```python
from build123d import *

# Parameters (mm, degrees)
F0_R     = 20
F1_DEPTH = 6
F2_R     = 5
F3_DEPTH = 12
F4_R     = 2.75
F5_DEPTH = 18.001
F6_R     = 5
F7_DEPTH = 5


with BuildPart() as f1:
    # F0 (on Top) → F1 (new body)
    with BuildSketch(Plane.XY):
        Circle(F0_R)
    extrude(amount=F1_DEPTH)

    # F2 (on face) → F3 (join)
    with BuildSketch(Plane.XY.offset(6)):
        Circle(F2_R)
    extrude(amount=F3_DEPTH)

    # F4 (on face) → F5 (cut, through all)
    with BuildSketch(Plane.XY.offset(18)):
        Circle(F4_R)
    extrude(amount=-F5_DEPTH, mode=Mode.SUBTRACT)

    # F6 (on face) → F7 (cut)
    with BuildSketch(Plane.XY):
        Circle(F6_R)
    extrude(amount=F7_DEPTH, mode=Mode.SUBTRACT)


solid = f1.part
```
Check sheet for the modelled part. Datum: model origin and axes. Units: mm. A direction names the side the tool comes from. Coordinates: 2 decimals unless noted, no trailing zeros. Write each loop counter-clockwise with the first axis right and the second up, starting at its lowest first coordinate (ties: lowest second). Pieces come first, ordered by that corner, then holes. Notation, with made-up numbers: M 3.5,34.25 L 50.5,34.25 A21 cw 50.5,43.25 Z; hole C 66,-9 d7. An arc over 180 degrees is marked long. Write item = value, one per line. Start each with the question number.
1. Mould release check, pull along Y, two halves, no side actions. Record for faces 3 (the flat face through (2.2, -2.2, 18)), 4 (the cylindrical face through (-1.08, -4.88, 2.46)), 5 (the cylindrical face through (-1.08, -4.88, 11.92)), 6 (the flat face through (2.2, -2.2, 5)): pulls with the +Y half, pulls with the -Y half, needs draft (parallel to the pull), parting line crosses it, or undercut.
2. Thickness scan on probe 1 along Y at (x, z) = (0, 3.5); probe 2 along Z at (x, y) = (-10, -3.5); probe 3 along Y at (x, z) = (0, 14.75). Record the ranges inside material, lowest first.
3. Go/stop test with flat-tipped pins: pin 1 (8 mm diameter, centred on x = -15.5, z = 2.5, fed in from +Y); pin 2 (5 mm diameter, centred on x = -3.5, z = 11.5, fed in from +Y); pin 3 (10 mm diameter, centred on y = 1.5, z = 16, fed in from +X). Record where each tip stops, or that it passes through.
4. Sectioned sample at A-A (x = 0). Record the cut outline in (y, z).
5. Sectioned sample at C-C (z = 13.5). Record the cut outline in (x, y), then the cut area to 3 significant figures.
6. Tool access check on faces 1 (the cylindrical face through (-4.336, -19.524, 2.958)), 2 (the flat face through (4, -4, 6)). Record the directions out of +Z, -Z, +X, -X, +Y, -Y that give a thin tool (end or side, any length) a straight path to the whole face; none if there is none.
7. Sectioned sample at D-D (y = -12). Record the cut outline in (x, z), then the cut area to 3 significant figures.
The answers:
q1.face_3 = needs draft
q1.face_4 = undercut
q1.face_5 = parting line crosses it
q1.face_6 = undercut
q2.probe_1 = -20 to -5, 5 to 20
q2.probe_2 = 0 to 6
q2.probe_3 = -5 to -2.75, 2.75 to 5
q3.pin_1 = 16.36
q3.pin_2 = 4.9
q3.pin_3 = 5
q4.outline = M -20,0 L -5,0 L -5,5 L -2.75,5 L -2.75,18 L -5,18 L -5,6 L -20,6 Z; M 2.75,5 L 5,5 L 5,0 L 20,0 L 20,6 L 5,6 L 5,18 L 2.75,18 Z
q5.outline = C 0,0 d10; hole C 0,0 d5.5
q5.area = 54.8 mm²
q6.face_1 = +Z, -Z
q6.face_2 = +Z
q7.outline = M -16,0 L 16,0 L 16,6 L -16,6 Z
q7.area = 192 mm²
